Part model, mm, in its own coordinate system. Face numbers are marked on the shaded views. A direction names the side the tool comes from. Give positions to 0.01 mm unless a question says otherwise; leave off trailing zeros. Write each loop counter-clockwise with the first axis right and the second up, starting at its lowest first coordinate (ties: lowest second). Pieces come first, ordered by that corner, then holes. Notation, with made-up numbers: (25.5, 43) - (41.5, 43) arc R20 cw to (41.5, 73) - close; hole circle Ø6 at (84.5, -28.5). An arc over 180 degrees is marked (long way). Answer in a Markdown table with one row per item. Add a question column.
1. Band-saw the part on D-D on y = 127. Write the cut outline in (x, z).
2. Probe line 1 along X through (y, z) = (8.5, -98); line 2 along Y through (x, z) = (71, 87); line 3 along X through (y, z) = (110, -38.5). List the from-to ranges inside material, lowest first.
3. Band-saw the part on A-A on z = -98. Write the cut outline in (x, y), plus the area to 3 significant figures.
4. Band-saw the part on B-B on x = 0. Write the cut outline in (y, z), plus the area to 3 significant figures.
5. Which spindle directions (+Z, -Z, +X, -X, +Y, -Y) get a long thin tool onto all of the face, cutting with end or side? Do the marked faces 1, 2, 3, 4 and 5. Say none if no direction does.
6. Drop flat-ended pins along their axis: pin 1 Ø12 at (x, y) = (-43.5, 138) entering from -Z; pin 2 Ø1 at (x, y) = (41, 91) entering from +Z; pin 3 Ø3 at (x, y) = (54, 46) entering from -Z. Give the stop position or say it passes through.
7. Band-saw the part on C-C on z = 0. Write the cut outline in (x, y).
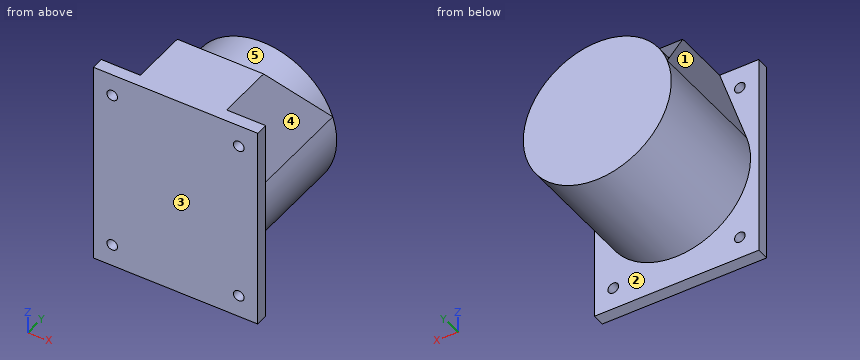
```python
from build123d import *

# Parameters (mm, degrees)
SKETCH1_W               = 250
SKETCH1_H               = 200
SKETCH1_R               = 6.5
BOSS_EXTRUDE1_DEPTH     = 15
BOSS_EXTRUDE2_DEPTH     = 150
CUT_EXTRUDE1_DEPTH      = 101
CUT_EXTRUDE1_DEPTH_BACK = 101
BOSS_EXTRUDE3_REACH     = 167
BODY_MOVE_COPY1_ANGLE   = 90


with BuildPart() as part:
    # Sketch1 → Boss-Extrude1 (new body)
    with BuildSketch(Plane(origin=(0, 0, 0), x_dir=(1, 0, 0), z_dir=(0, 1, 0))):
        Rectangle(SKETCH1_W, SKETCH1_H)
        with Locations((-98, 77)):
            Circle(SKETCH1_R, mode=Mode.SUBTRACT)
        with Locations((98, 77)):
            Circle(SKETCH1_R, mode=Mode.SUBTRACT)
        with Locations((-98, -77)):
            Circle(SKETCH1_R, mode=Mode.SUBTRACT)
        with Locations((98, -77)):
            Circle(SKETCH1_R, mode=Mode.SUBTRACT)
    extrude(amount=BOSS_EXTRUDE1_DEPTH)

    # Sketch2 → Boss-Extrude2 (add)
    with BuildSketch(Plane(origin=(0, 15, 0), x_dir=(1, 0, 0), z_dir=(0, 1, 0))):
        with BuildLine():
            Line((125, 52.5), (29.018785036, 85.193368962))
            ThreePointArc((29.018785036, 85.193368962), (-90, 0), (29.018785036, -85.193368962))
            Line((29.018785036, -85.193368962), (125, -52.5))
            Line((125, -52.5), (125, 52.5))
        make_face()
    extrude(amount=BOSS_EXTRUDE2_DEPTH)

    # Sketch3 → Cut-Extrude1 (cut, two sides)
    with BuildSketch(Plane.XY) as cut_extrude1_sk:
        Polygon((-384.335484925, 509.529308254), (29.018785036, 165), (125, 85), (538.354269961, -259.529308254), (1227.412886469, 567.179231668), (304.723131583, 1336.237848176), align=None)
    extrude(amount=CUT_EXTRUDE1_DEPTH, mode=Mode.SUBTRACT)
    extrude(cut_extrude1_sk.sketch, amount=-CUT_EXTRUDE1_DEPTH_BACK, mode=Mode.SUBTRACT)

    # Sketch4 → Boss-Extrude3 (add, up to next)
    with BuildSketch(Plane(origin=(0, 165, 0), x_dir=(1, 0, 0), z_dir=(0, 1, 0)), mode=Mode.PRIVATE) as boss_extrude3_sk1:
        with BuildLine():
            Line((29.018785036, -85.193368962), (29.018785036, 85.193368962))
            ThreePointArc((29.018785036, 85.193368962), (90, 0), (29.018785036, -85.193368962))
        make_face()
    boss_extrude3_tool1 = extrude(boss_extrude3_sk1.sketch, amount=-BOSS_EXTRUDE3_REACH, mode=Mode.PRIVATE) - part.part
    add(boss_extrude3_tool1.solids().sort_by_distance((54.295969, 165, 0))[0])


with BuildPart() as part_1:
    # Body-Move/Copy1: moved
    add(part.part.rotate(Axis((0, 0, 0), (0, -1, 0)), BODY_MOVE_COPY1_ANGLE))


solid = part_1.part
```
Values:
| question | item | result |
|---|---|---|
| 1 | outline | (-85.19, 29.02) arc R90 ccw (long way) to (85.19, 29.02) - (69.66, 74.61) - (50.33, 74.61) arc R90 ccw to (-50.33, 74.61) - (-69.66, 74.61) - close |
| 2 | line 1 | x = -100 to -83.5, -70.5 to 70.5, 83.5 to 100 |
| 2 | line 2 | y = 0 to 15 |
| 2 | line 3 | x = -81.35 to 81.35 |
| 3 | outline | (-100, 0) - (-83.5, 0) - (-83.5, 15) - (-100, 15) - close; (-70.5, 0) - (70.5, 0) - (70.5, 15) - (-70.5, 15) - close; (83.5, 0) - (100, 0) - (100, 15) - (83.5, 15) - close |
| 3 | area | 2,610 mm² |
| 4 | outline | (0, -125) - (15, -125) - (15, -90) - (165, -90) - (165, 90) - (114.17, 90) - (85, 125) - (0, 125) - close |
| 4 | area | 33,700 mm² |
| 5 | face 1 | +Z, -X, +Y |
| 5 | face 2 | +Y |
| 5 | face 3 | +Z, -Z, +X, -X, -Y |
| 5 | face 4 | +Z, +X, +Y |
| 5 | face 5 | +Z, +Y |
| 6 | pin 1 | stops at z = -81.82 |
| 6 | pin 2 | stops at z = 118.4 |
| 6 | pin 3 | stops at z = -73.1 |
| 7 | outline | (-100, 0) - (100, 0) - (100, 15) - (90, 15) - (90, 165) - (-90, 165) - (-90, 15) - (-100, 15) - close |
